```python
from build123d import *

# Parameters (mm, degrees)
ESQUISSE1_W        = 250
ESQUISSE1_H        = 40
BOSS_EXTRU_1_DEPTH = 5
BOSS_EXTRU_2_DEPTH = 250


with BuildPart() as part:
    # Esquisse1 → Boss.-Extru.1 (new body)
    with BuildSketch(Plane.XY):
        with Locations((125, 20)):
            Rectangle(ESQUISSE1_W, ESQUISSE1_H)
    extrude(amount=BOSS_EXTRU_1_DEPTH)

    # Esquisse2 → Boss.-Extru.2 (add)
    with BuildSketch(Plane.ZY):
        Polygon((0, 0), (-10, 0), (0, 2.320632566), align=None)
    extrude(amount=-BOSS_EXTRU_2_DEPTH)


solid = part.part
```
Build history of the part. All positions in model axes, mm. A direction names the side the tool comes from. Coordinates: 2 decimals unless noted, no trailing zeros. Order: outer loops, then holes, each group sorted by start corner. A loop starts at its lowest first (then second) coordinate and runs counter-clockwise, first axis right, second up. Notation, with made-up numbers: (8, 81) -> (27, 81) arc R12 ccw to (27, 101) -> close; hole circle Ø11 at (-10, 6). An arc over 180 degrees is marked (long way). Answer in a Markdown table with one row per item. Add a question column.
Q1. Band-saw the part on B-B, the plane y = 23. List the corners of the cut face in (x, z).
Q2. Which spindle directions (+Z, -Z, +X, -X, +Y, -Y) get a long thin tool onto all of the face, cutting with end or side? Do faces 1 (the face through (123, 21, 0)), 2 (the face through (0, 19, 1)). Say none if no direction does.
Q3. Wall check: line 1 along Z through (x, y) = (121.5, 16); line 2 along Y through (x, z) = (46.5, -1); line 3 along Y through (x, z) = (36, -4.75). Give the ranges that are in metal, low to high. Write a range as [from, to].
Q4. Band-saw the part on A-A, the plane x = 56. List the corners of the cut face in (y, z).
Q5. Band-saw the part on C-C, the plane z = -2.5. List the corners of the cut face in (x, y).
Q6. Drop flat-ended pins along their axis: pin 1 (8 mm diameter, centred on y = 7.5, z = -7.5, fed in from -X); pin 2 (8 mm diameter, centred on x = 174.5, y = 32.5, fed in from -Z). Give the stop position or say it passes through.
Answers follow:
| question | item | result |
|---|---|---|
| 1 | outline | (0, 0) -> (250, 0) -> (250, 5) -> (0, 5) -> close |
| 2 | face 1 | -Z, +X, -X, +Y |
| 2 | face 2 | +Z, -Z, -X, +Y, -Y |
| 3 | line 1 | [0, 5] |
| 3 | line 2 | [0, 2.09] |
| 3 | line 3 | [0, 1.22] |
| 4 | outline | (0, -10) -> (2.32, 0) -> (40, 0) -> (40, 5) -> (0, 5) -> close |
| 5 | outline | (0, 0) -> (250, 0) -> (250, 1.74) -> (0, 1.74) -> close |
| 6 | pin 1 | through |
| 6 | pin 2 | z = 0 |
